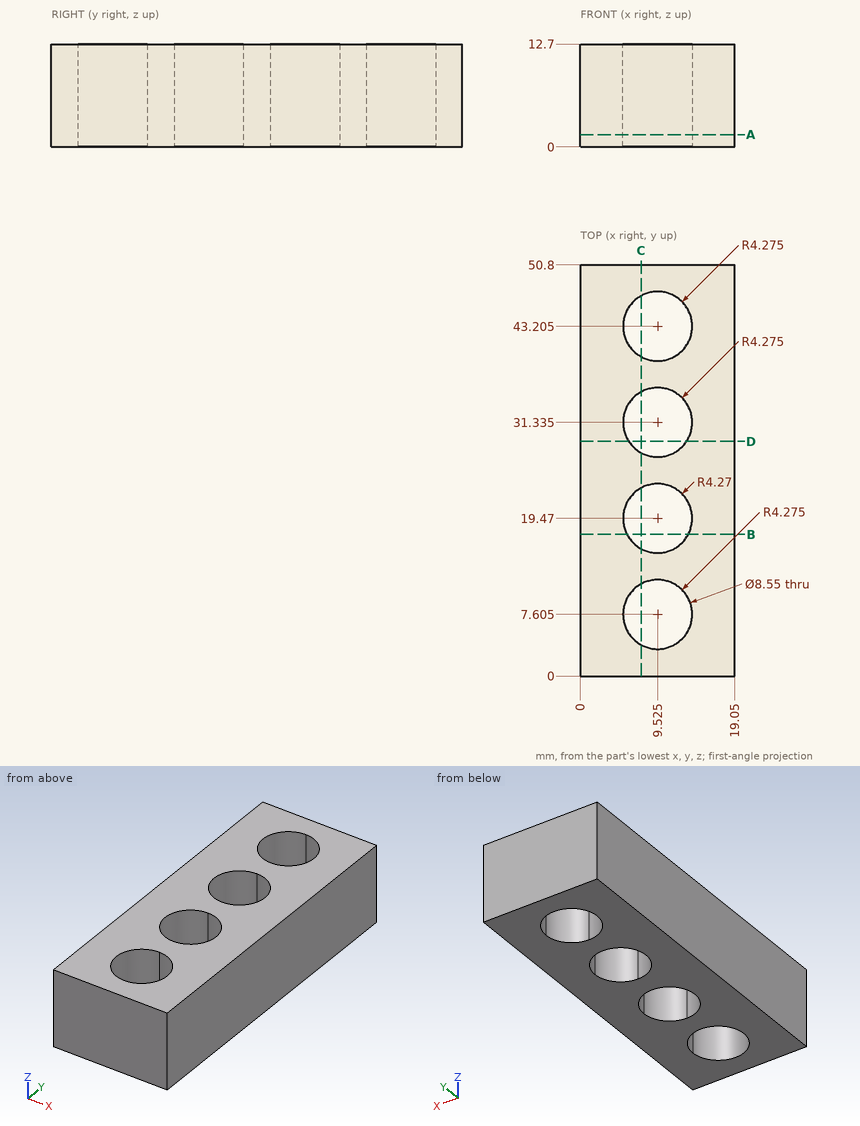
Design review of the part shown in the three views and the two pictorial views. Dimensions are in mm from the part's minimum x, y and z. Give positions to 0.01 mm unless a question says otherwise; leave off trailing zeros. Loops run counter-clockwise (first coordinate to the right, second up) from the corner with the lowest first, then second, coordinate; pieces in that order, holes last. Notation, with made-up numbers: (-5, 8.5) -> (53, 8.5) arc R26 ccw to (53, 33.5) -> close; hole circle Ø10 at (22, 59.5). An arc over 180 degrees is marked (long way). Put each result on its own line as item: value. Start each with the question number.
1. We need section A-A on z = 1.5. State the section outline as (x, y) points (3 decimals).
2. We need section B-B on y = 17.5. State the section outline as (x, z) points, then the cut area to 3 significant figures.
3. We need section C-C on x = 7.5. State the section outline as (y, z) points, then the cut area to 3 significant figures.
4. Clearance check with a flat-ended pin moving along its axis: P1, Ø1.5, axis at x = 11, y = 10.5, coming from the -Z side. State where the tip first meets the part, or that it passes through.
5. Wall thickness on probe 1 along Y at (x, z) = (9.25, 3); probe 2 along Y at (x, z) = (10.5, 4); probe 3 along X at (y, z) = (10, 6.5): over which ranges is each line inside the solid? List them lowest first.
6. We need section D-D on y = 29. State the section outline as (x, z) points, then the cut area to 3 significant figures.
Determined:
1. outline: (0, 0) -> (19.05, 0) -> (19.05, 50.8) -> (0, 50.8) -> close; hole circle Ø8.55 at (9.525, 7.605); hole circle Ø8.55 at (9.525, 31.335); hole circle Ø8.55 at (9.525, 43.205); hole circle Ø8.54 at (9.525, 19.47)
2. outline: (0, 0) -> (5.74, 0) -> (5.74, 12.7) -> (0, 12.7) -> close; (13.31, 0) -> (19.05, 0) -> (19.05, 12.7) -> (13.31, 12.7) -> close
2. area: 146 mm^2
3. outline: (0, 0) -> (3.84, 0) -> (3.84, 12.7) -> (0, 12.7) -> close; (11.37, 0) -> (15.71, 0) -> (15.71, 12.7) -> (11.37, 12.7) -> close; (23.23, 0) -> (27.57, 0) -> (27.57, 12.7) -> (23.23, 12.7) -> close; (35.1, 0) -> (39.44, 0) -> (39.44, 12.7) -> (35.1, 12.7) -> close; (46.97, 0) -> (50.8, 0) -> (50.8, 12.7) -> (46.97, 12.7) -> close
3. area: 263 mm^2
4. P1: through
5. probe 1: 0 to 3.34, 11.87 to 15.21, 23.73 to 27.07, 35.6 to 38.94, 47.47 to 50.8
5. probe 2: 0 to 3.44, 11.77 to 15.31, 23.63 to 27.17, 35.5 to 39.04, 47.37 to 50.8
5. probe 3: 0 to 5.98, 13.07 to 19.05
6. outline: (0, 0) -> (5.94, 0) -> (5.94, 12.7) -> (0, 12.7) -> close; (13.11, 0) -> (19.05, 0) -> (19.05, 12.7) -> (13.11, 12.7) -> close
6. area: 151 mm^2
